Source: CAD feature listing. Evaluate the final solid. Frame: model axes, mm. A direction names the side the tool comes from. Coordinates: 2 decimals unless noted, no trailing zeros. Write each loop counter-clockwise with the first axis right and the second up, starting at its lowest first coordinate (ties: lowest second). Pieces come first, ordered by that corner, then holes. Notation, with made-up numbers: (46, 67) - (67, 67) arc R26 ccw to (67, 93) - close; hole circle Ø10 at (27, 56.25). An arc over 180 degrees is marked (long way). One line per question, with ' | ' between items.
from build123d import *

# Parameters (mm, degrees)
BOX005_W     = 15
BOX005_H     = 5
BOX005_DEPTH = 16
BOX004_W     = 15
BOX004_H     = 5
BOX004_DEPTH = 16
BOX_W        = 120
BOX_H        = 280
BOX_DEPTH    = 5


with BuildPart() as cubo004:
    # Box005 → Box005 (new body)
    with BuildSketch(Plane(origin=(35, 82, 69), x_dir=(1, 0, 0), z_dir=(0, 0, 1))):
        with Locations((7.5, 2.5)):
            Rectangle(BOX005_W, BOX005_H)
    extrude(amount=BOX005_DEPTH)


with BuildPart() as cubo003:
    # Box004 → Box004 (new body)
    with BuildSketch(Plane(origin=(35, -87, 68), x_dir=(1, 0, 0), z_dir=(0, 0, 1))):
        with Locations((7.5, 2.5)):
            Rectangle(BOX004_W, BOX004_H)
    extrude(amount=BOX004_DEPTH)


with BuildPart() as obj1:
    # Box → Box (new body)
    with BuildSketch(Plane(origin=(-6, -140, 73.5), x_dir=(1, 0, 0), z_dir=(0, 0, 1))):
        with Locations((60, 140)):
            Rectangle(BOX_W, BOX_H)
    extrude(amount=BOX_DEPTH)

    # Cut003: cut Cubo003
    add(cubo003.part, mode=Mode.SUBTRACT)

    # Cut004: cut Cubo004
    add(cubo004.part, mode=Mode.SUBTRACT)


with BuildPart() as obj1_1:
    # Cut004 placement: moved
    add(obj1.part.moved(Location((0, 0, -70))))


solid = obj1_1.part
Item 1: Mould query, pull axis X, two halves, no side actions, for faces 1 (the face through (53, 2, 8.5)), 2 (the face through (42, -82, 6)), 3 (the face through (-6, -2, 6)). Classes: pulls with the +X half, pulls with the -X half, needs draft (parallel to the pull), parting line crosses it, or undercut.
Check sheet entries:
face 1: needs draft | face 2: undercut | face 3: pulls with the -X half
Item 2: Ray query, line 1 along Y through (x, z) = (36.5, 4.85). Return the intervals inside material, ascending. Write a range as [from, to].
Check sheet entries:
line 1: [-140, -87], [-82, 82], [87, 140]
Item 3: Cut plane A-A on x = 45. Return loops of the section in (y, z).
Check sheet entries:
outline: (-140, 3.5) - (-87, 3.5) - (-87, 8.5) - (-140, 8.5) - close; (-82, 3.5) - (82, 3.5) - (82, 8.5) - (-82, 8.5) - close; (87, 3.5) - (140, 3.5) - (140, 8.5) - (87, 8.5) - close
Item 4: Access query for faces 4 (the face through (50, -85, 6)), 5 (the face through (53, 140, 6)). Directions: +Z, -Z, +X, -X, +Y, -Y. A direction counts if a zero-diameter tool reaches every point of the face in a straight line with its end or side. Return the directions, or none.
Check sheet entries:
face 4: +Z, -Z | face 5: +Z, -Z, +X, -X, +Y
